```python
from build123d import *

# Parameters (mm, degrees)
SKETCH1_W           = 609.6
SKETCH1_H           = 387.4
BOSS_EXTRUDE1_DEPTH = 76.2
SKETCH2_W           = 573.6
SKETCH2_H           = 351.4
CUT_EXTRUDE1_DEPTH  = 25.4
SKETCH3_W           = 50.8
SKETCH3_H           = 54.95
CUT_EXTRUDE2_DEPTH  = 35.8
BOSS_EXTRUDE2_DEPTH = 25.4


with BuildPart() as part:
    # Sketch1 → Boss-Extrude1 (new body)
    with BuildSketch(Plane(origin=(0, 0, 0), x_dir=(1, 0, 0), z_dir=(0, 1, 0))):
        with Locations((32.357180973, 74.716472916)):
            Rectangle(SKETCH1_W, SKETCH1_H)
    extrude(amount=-BOSS_EXTRUDE1_DEPTH)

    # Sketch2 → Cut-Extrude1 (cut)
    with BuildSketch(Plane(origin=(0, 0, 0), x_dir=(1, 0, 0), z_dir=(0, 1, 0))):
        with Locations((32.357180973, 74.716472916)):
            Rectangle(SKETCH2_W, SKETCH2_H)
    extrude(amount=-CUT_EXTRUDE1_DEPTH, mode=Mode.SUBTRACT)

    # Sketch3 → Cut-Extrude2 (cut)
    with BuildSketch(Plane(origin=(0, -25.4, 0), x_dir=(1, 0, 0), z_dir=(0, 1, 0))):
        with Locations((293.757180973, 172.141472916)):
            Rectangle(SKETCH3_W, SKETCH3_H)
        with Locations((293.757180973, 107.191472916)):
            Rectangle(SKETCH3_W, SKETCH3_H)
        with Locations((293.757180973, 42.241472916)):
            Rectangle(SKETCH3_W, SKETCH3_H)
        with Locations((293.757180973, -22.708527084)):
            Rectangle(SKETCH3_W, SKETCH3_H)
    extrude(amount=-CUT_EXTRUDE2_DEPTH, mode=Mode.SUBTRACT)

    # Sketch7 → Boss-Extrude2 (add)
    with BuildSketch(Plane(origin=(0, -25.4, 0), x_dir=(1, 0, 0), z_dir=(0, 1, 0))):
        Polygon((319.157180973, 209.616472916), (258.357180973, 209.616472916), (258.357180973, -60.183527084), (319.157180973, -60.183527084), (319.157180973, -50.183527084), (268.357180973, -50.183527084), (268.357180973, 4.766472916), (319.157180973, 4.766472916), (319.157180973, 14.766472916), (268.357180973, 14.766472916), (268.357180973, 69.716472916), (319.157180973, 69.716472916), (319.157180973, 79.716472916), (268.357180973, 79.716472916), (268.357180973, 134.666472916), (319.157180973, 134.666472916), (319.157180973, 144.666472916), (268.357180973, 144.666472916), (268.357180973, 199.616472916), (319.157180973, 199.616472916), align=None)
    extrude(amount=BOSS_EXTRUDE2_DEPTH)


solid = part.part
```
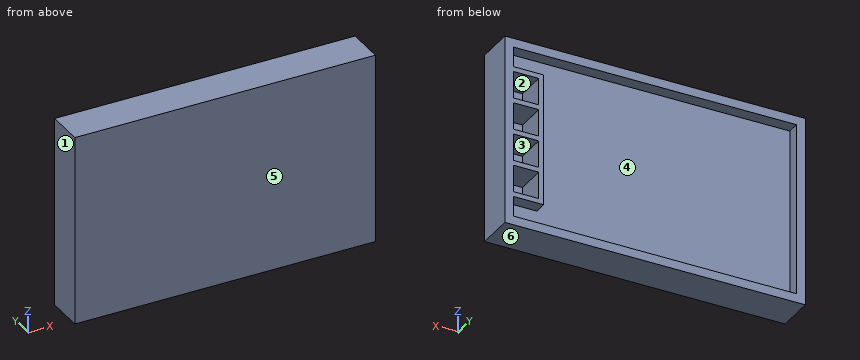
The listing builds one solid part. Answer for the finished solid, in the listing's coordinates (mm). Face numbers are marked on the shaded views. A direction names the side the tool comes from. Coordinates: 2 decimals unless noted, no trailing zeros. Write each loop counter-clockwise with the first axis right and the second up, starting at its lowest first coordinate (ties: lowest second). Pieces come first, ordered by that corner, then holes. Notation, with made-up numbers: (-11, 35) -> (28, 35) arc R8 ccw to (28, 39) -> close; hole circle Ø7 at (65, -22.5). An arc over 180 degrees is marked (long way). Write each question's results on one line, items separated by ' | '. Start each with the question number.
1) A tool of negligible diameter and unlimited length cuts with its end or side. For the marked faces 1 and 2, from which of +Z, -Z, +X, -X, +Y, -Y can it reach the whole face along a straight path? Write none if from no direction.
2) For a pull along Z with two mould halves and no side action, classify the marked faces 3, 4, 5 and 6 as +Z half, -Z half, draft (parallel to the pull), parting line (faces both ways), or undercut.
3) A cutting plane is placed at D-D (y = -15.5). Determine the outline of the cut face in (x, z).
4) A cutting plane is placed at A-A (y = -52). Determine the outline of the cut face in (x, z), then the cut area to 3 significant figures.
5) A cutting plane is placed at B-B (z = -61.5). Determine the outline of the cut face in (x, y), then the cut area to 3 significant figures.
6) A flat-ended cylindrical pin translates along its axis: pin 1 Ø15 at (x, z) = (299, 20) entering from +Y. Find the tip coordinate at first contact, or state that the pin passes through.
7) Straight lines are drawn through the part: probe 1 along X at (y, z) = (-23, -56); probe 2 along Z at (x, y) = (169.5, -14); probe 3 along X at (y, z) = (-58, -178). For each, find the intervals that lie inside material, in ascending order.
8) A cutting plane is placed at C-C (x = 113.5). Determine the outline of the cut face in (y, z).
Values follow:
1) face 1: +Z, -Z, -X, +Y, -Y | face 2: +Y
2) face 3: undercut | face 4: undercut | face 5: draft | face 6: -Z half
3) outline: (-272.44, -268.42) -> (337.16, -268.42) -> (337.16, 118.98) -> (-272.44, 118.98) -> close; hole (-254.44, -250.42) -> (319.16, -250.42) -> (319.16, -209.62) -> (258.36, -209.62) -> (258.36, 60.18) -> (319.16, 60.18) -> (319.16, 100.98) -> (-254.44, 100.98) -> close; hole (268.36, -199.62) -> (319.16, -199.62) -> (319.16, -144.67) -> (268.36, -144.67) -> close; hole (268.36, -134.67) -> (319.16, -134.67) -> (319.16, -79.72) -> (268.36, -79.72) -> close; hole (268.36, -69.72) -> (319.16, -69.72) -> (319.16, -14.77) -> (268.36, -14.77) -> close; hole (268.36, -4.77) -> (319.16, -4.77) -> (319.16, 50.18) -> (268.36, 50.18) -> close
4) outline: (-272.44, -268.42) -> (337.16, -268.42) -> (337.16, 118.98) -> (-272.44, 118.98) -> close; hole (268.36, -199.62) -> (319.16, -199.62) -> (319.16, -144.67) -> (268.36, -144.67) -> close; hole (268.36, -134.67) -> (319.16, -134.67) -> (319.16, -79.72) -> (268.36, -79.72) -> close; hole (268.36, -69.72) -> (319.16, -69.72) -> (319.16, -14.77) -> (268.36, -14.77) -> close; hole (268.36, -4.77) -> (319.16, -4.77) -> (319.16, 50.18) -> (268.36, 50.18) -> close | area: 225,000 mm²
5) outline: (-272.44, -76.2) -> (337.16, -76.2) -> (337.16, 0) -> (319.16, 0) -> (319.16, -61.2) -> (268.36, -61.2) -> (268.36, 0) -> (258.36, 0) -> (258.36, -25.4) -> (-254.44, -25.4) -> (-254.44, 0) -> (-272.44, 0) -> close | area: 30,300 mm²
6) pin 1: y = -61.2
7) probe 1: -272.44 to -254.44, 258.36 to 268.36, 319.16 to 337.16 | probe 2: -268.42 to -250.42, 100.98 to 118.98 | probe 3: -272.44 to 268.36, 319.16 to 337.16
8) outline: (-76.2, -268.42) -> (0, -268.42) -> (0, -250.42) -> (-25.4, -250.42) -> (-25.4, 100.98) -> (0, 100.98) -> (0, 118.98) -> (-76.2, 118.98) -> close
